```python
from build123d import *

# Parameters (mm, degrees)
SKETCH1_W           = 45.72
SKETCH1_H           = 25.4
BOSS_EXTRUDE1_DEPTH = 4
SKETCH2_W           = 3
SKETCH2_H           = 25.4
BOSS_EXTRUDE2_DEPTH = 20
CHAMFER1_SIZE       = 5
BOSS_EXTRUDE3_DEPTH = 4
SKETCH4_R           = 1.75
CUT_EXTRUDE1_DEPTH  = 4
SKETCH5_R           = 1.75
CUT_EXTRUDE2_DEPTH  = 14
FILLET1_R           = 3


with BuildPart() as part:
    # Sketch1 → Boss-Extrude1 (new body)
    with BuildSketch(Plane(origin=(0, 0, 0), x_dir=(1, 0, 0), z_dir=(0, 1, 0))):
        Rectangle(SKETCH1_W, SKETCH1_H)
    extrude(amount=BOSS_EXTRUDE1_DEPTH)

    # Sketch2 → Boss-Extrude2 (add)
    with BuildSketch(Plane(origin=(0, 4, 0), x_dir=(1, 0, 0), z_dir=(0, 1, 0))):
        with Locations((-2.3, 0)):
            Rectangle(SKETCH2_W, SKETCH2_H)
        with Locations((2.3, 0)):
            Rectangle(SKETCH2_W, SKETCH2_H)
    extrude(amount=BOSS_EXTRUDE2_DEPTH)

    # Chamfer1
    chamfer1_edges = [part.edges().sort_by_distance(p)[0] for p in [
        (-3.8, 4, 0),
        (3.8, 4, 0),
    ]]
    chamfer(chamfer1_edges, length=CHAMFER1_SIZE)

    # Sketch3 → Boss-Extrude3 (add)
    with BuildSketch(Plane(origin=(0, 0, -12.7), x_dir=(-1, 0, 0), z_dir=(0, 0, -1))):
        Polygon((-3.8, 24), (-22.86, 4), (-3.8, 4), align=None)
        Polygon((3.8, 24), (3.8, 4), (22.86, 4), align=None)
    extrude(amount=-BOSS_EXTRUDE3_DEPTH)

    # Sketch4 → Cut-Extrude1 (cut)
    with BuildSketch(Plane.XZ):
        with Locations(Location((-12.7, 0, 0), (0, 0, 270))):
            Circle(SKETCH4_R)
        with Locations(Location((12.7, 0, 0), (0, 0, 270))):
            Circle(SKETCH4_R)
    extrude(amount=-CUT_EXTRUDE1_DEPTH, mode=Mode.SUBTRACT)

    # Sketch5 → Cut-Extrude2 (cut)
    with BuildSketch(Plane.ZY.offset(3.8)):
        with Locations((0, 11)):
            Circle(SKETCH5_R)
    extrude(amount=-CUT_EXTRUDE2_DEPTH, mode=Mode.SUBTRACT)

    # Fillet1
    fillet1_edges = [part.edges().sort_by_distance(p)[0] for p in [
        (-2.3, 24, 12.7),
        (2.3, 24, 12.7),
        (22.86, 2, 12.7),
        (-22.86, 2, 12.7),
        (-22.86, 2, -12.7),
        (22.86, 2, -12.7),
    ]]
    fillet(fillet1_edges, radius=FILLET1_R)


solid = part.part
```
The listing builds one solid part. Answer for the finished solid, in the listing's coordinates (mm). A direction names the side the tool comes from. Round coordinates to 2 decimals unless told otherwise and drop trailing zeros. Loops run counter-clockwise (first coordinate to the right, second up) from the corner with the lowest first, then second, coordinate; pieces in that order, holes last. Notation, with made-up numbers: (11.5, 48.5) - (42.5, 48.5) arc R13 cw to (42.5, 72.5) - close; hole circle Ø4 at (16.25, 34.25). An arc over 180 degrees is marked (long way). Return JSON: item names as keys, results as strings. Group by question number.
1. The part is cut by section B-B on x = -1.5. Determine the outline of the cut face in (y, z), then the cut area to 3 significant figures.
2. Consider probe 1 along X at (y, z) = (2.95, 0); probe 2 along Y at (x, z) = (-1.85, 0); probe 3 along X at (y, z) = (23, -0.75). Determine where each line is inside the solid, lowest interval first.
3. Each of these flat-tipped pins is pushed along its axis until it touches: P1, Ø6, axis at y = 15, z = -4, coming from the -X side; P2, Ø4, axis at x = -12.7, z = 0, coming from the +Y side; P3, Ø4.5, axis at y = 13.5, z = 5, coming from the +X side; P4, Ø3, axis at y = 11, z = 0, coming from the +X side. Where does it stop, or does it pass through?
4. The mould has two halves that part along Z. Classify faces 1 (the cylindrical face through (2.32, 23.14, 11.8)), 2 (the cylindrical face through (2.279, 12.735, -0.228)), 3 (the flat face through (0, 0, 0)): pulls with the +Z half, pulls with the -Z half, needs draft (parallel to the pull), parting line crosses it, or undercut.
5. The part is cut by section A-A on z = 0. State how many separate pieces and enclosed holes the cut face has, then the cut area to 3 significant figures.
6. The part is cut by section D-D on y = 11. Determine the outline of the cut face in (x, z).
7. Which of the six approach directions +Z, -Z, +X, -X, +Y, -Y give full straight-line access (tool end or side, diameter ignored) to faces 4 (the flat face through (0, 4, 0)), 5 (the flat face through (11, 12, -8.7)), 6 (the flat face through (-6.3, 6.5, 2.1))?
8. The part is cut by section C-C on y = 2.5. Determine the outline of the cut face in (x, z).
Resolved:
{
 "1": {"outline": "(0, -12.7) - (24, -12.7) - (24, 9.7) arc R3 ccw to (21, 12.7) - (0, 12.7) - close; hole circle Ø3.5 at (11, 0)", "area": "598 mm²"},
 "2": {"probe 1": "x = -22.86 to -14.45, -10.95 to 10.95, 14.45 to 22.86", "probe 2": "y = 0 to 9.25, 12.75 to 24", "probe 3": "x = -3.8 to -0.8, 0.8 to 3.8"},
 "3": {"P1": "stops at x = -3.8", "P2": "stops at y = 4", "P3": "stops at x = 3.8", "P4": "passes through"},
 "4": {"face 1": "pulls with the +Z half", "face 2": "undercut", "face 3": "needs draft"},
 "5": {"separate pieces": "5", "enclosed holes": "0", "area": "279 mm²"},
 "6": {"outline": "(-16.19, -12.7) - (-0.8, -12.7) - (-0.8, -1.75) - (-3.8, -1.75) - (-3.8, -8.7) - (-16.19, -8.7) - close; (-3.8, 1.75) - (-0.8, 1.75) - (-0.8, 12.7) - (-3.8, 12.7) - close; (0.8, -12.7) - (16.19, -12.7) - (16.19, -8.7) - (3.8, -8.7) - (3.8, -1.75) - (0.8, -1.75) - close; (0.8, 1.75) - (3.8, 1.75) - (3.8, 12.7) - (0.8, 12.7) - close"},
 "7": {"face 4": "+Z, -Z, +Y", "face 5": "+Z, +X, +Y", "face 6": "+Z, -X, +Y"},
 "8": {"outline": "(-22.86, -9.7) arc R3 ccw to (-19.86, -12.7) - (19.86, -12.7) arc R3 ccw to (22.86, -9.7) - (22.86, 9.7) arc R3 ccw to (19.86, 12.7) - (-19.86, 12.7) arc R3 ccw to (-22.86, 9.7) - close; hole circle Ø3.5 at (-12.7, 0); hole circle Ø3.5 at (12.7, 0)"}
}
